The listing builds one solid part. Answer for the finished solid, in the listing's coordinates (mm). A direction names the side the tool comes from. Coordinates: 2 decimals unless noted, no trailing zeros. Order: outer loops, then holes, each group sorted by start corner. A loop starts at its lowest first (then second) coordinate and runs counter-clockwise, first axis right, second up. Notation, with made-up numbers: (41.25, 83) -> (82.25, 83) arc R9 ccw to (82.25, 92) -> close; hole circle Ø3 at (78.5, 25). An arc over 180 degrees is marked (long way). Write item = value, one per line. Start each with the question number.
Autodesk Inventor part; units mm, degrees
ref_plane "Work Plane1" through (0, 0, -10) normal (0, 0, 1) x (1, 0, 0)
ref_plane "Work Plane2" through (0, 0, 0) normal (0.7071, -0.7071, 0) x (0, 0, -1)
ref_plane "YZ Plane" through (0, 0, 0) normal (1, 0, 0) x (0, 1, 0)
sketch "Sketch1" plane through (0, 0, 0) normal (0, 0, 1) x (1, 0, 0)
  line L0 (0, 0) -> (27.5, 0)
  line L1 (27.5, 0) -> (27.5, 5.5)
  line L2 (27.5, 5.5) -> (23, 5.5)
  line L3 (0, 0) -> (0, 27.5)
  line L4 (0, 0) -> (27.5, 0) construction
  line L5 (0, 27.5) -> (5.5, 27.5)
  line L6 (5.5, 27.5) -> (5.5, 23)
  line L7 (5.5, 23) -> (23, 5.5)
  dimension "d0" = 27.5
  dimension "d1" = 5.5
  dimension "d2" = 4.5
  dimension "d3" = 27.5
  dimension "d4" = 90
  dimension "d5" = 5.5
  dimension "d6" = 4.5
sketch "Sketch2" plane through (0, 0, 0) normal (0, 0, 1) x (1, 0, 0)
  line L0 (0, 0) -> (3.5, 0)
  line L1 (3.5, 3.5) -> (3.5, 27.5)
  line L2 (3.5, 27.5) -> (0, 27.5)
  line L3 (0, 27.5) -> (0, 0)
  line L4 (0, 0) -> (27.5, 0)
  line L5 (27.5, 0) -> (27.5, 3.5)
  line L6 (27.5, 3.5) -> (3.5, 3.5)
  line L7 (0, 3.5) -> (0, 0)
  dimension "d7" = 3.5
  dimension "d8" = 27.5
  dimension "d9" = 27.5
  dimension "d10" = 3.5
extrude "Extrusion1" add sketch "Sketch2" against normal blind 20
extrude "Extrusion2" add sketch "Sketch1" against normal blind 3.5
ref_plane "Work Plane1" through (0, 0, -10) normal (0, 0, 1) x (1, 0, 0)
mirror "Mirror1" about plane through (0, 0, -10) normal (0, 0, 1) of "Extrusion2"
sketch "Sketch3" plane through (0, 0, 0) normal (-1, 0, 0) x (0, 0, 1)
  line L0 (0, 0) -> (-20, 0) construction
  line L1 (-10, 0) -> (-10, 15) construction
  line L2 (-10, 14.8275) -> (-6.75, 14.8275) construction
  line L3 (-6.75, 14.8275) -> (-6.75, 9.8275) construction
  line L4 (-10, 9.8275) -> (-10, 14.8275) construction
  line L5 (-13.25, 13.0775) -> (-13.25, 17.1562)
  line L6 (-10, 20.4062) -> (-10, 20.4062)
  line L7 (-6.75, 17.1562) -> (-6.75, 13.0775)
  arc A0 (-10, 20.4062) -> (-13.25, 17.1562) centre (-10, 17.1562) ccw
  arc A1 (-6.75, 17.1562) -> (-10, 20.4062) centre (-10, 17.1562) ccw
  arc A2 (-13.25, 13.0775) -> (-10, 9.8275) centre (-10, 13.0775) ccw
  line L8 (-10, 9.8275) -> (-10, 9.8275)
  arc A3 (-10, 9.8275) -> (-6.75, 13.0775) centre (-10, 13.0775) ccw
  point P0 (-13.25, 20.4062)
  point P1 (-6.75, 20.4062)
  dimension "d16" = 15
  dimension "d17" = 3.25
  dimension "d18" = 5
  dimension "d19" = 6.5
  dimension "d20" = 3.25
  dimension "d21" = 3.25
extrude "Extrusion3" cut sketch "Sketch3" against normal through all
ref_plane "Work Plane2" through (0, 0, 0) normal (0.7071, -0.7071, 0) x (0, 0, -1)
mirror "Mirror2" about plane through (0, 0, 0) normal (0.7071, -0.7071, 0) of "Extrusion3"
properties part number "bracket"
Item 1: Consider probe 1 along Z at (x, y) = (4.5, 15.25); probe 2 along X at (y, z) = (25.75, -8.5). Determine where each line is inside the solid, lowest interval first.
Item 2: Section C-C, the plane x = 8.5 is taken. Give the vertices of the cut face in (y, z), then the cut area to 4 significant figures.
Item 3: Section B-B, the plane y = 16 is taken. Give the vertices of the cut face in (x, z).
Item 4: Each of these flat-tipped pins is pushed along its axis until it touches: pin 1 (6 mm diameter, centred on y = 9, z = -11.5, fed in from +X); pin 2 (5 mm diameter, centred on x = 9, z = -8.5, fed in from +Y); pin 3 (1.8 mm diameter, centred on x = 26, z = -19, fed in from +Y). Where does it stop, or does it pass through?
Item 5: Which of the six approach directions +Z, -Z, +X, -X, +Y, -Y give full straight-line access (tool end or side, diameter ignored) to faces 1 (the flat face through (5.5, 25, -2)), 2 (the flat face through (11, 11, 0)), 3 (the flat face through (10, 10, -3.5)), 4 (the cylindrical face through (1.73, 9.83, -10.07)), 5 (the flat face through (15, 2, -6.75))?
Item 6: Section D-D, the plane y = 23.75 is taken. Give the vertices of the cut face in (x, z), then the cut area to 3 significant figures.
Item 7: For a pull along Y with two mould halves and no side action, classify faces 6 (the flat face through (16, 3.5, -6)), 7 (the flat face through (2, 15, -6.75)), 8 (the flat face through (11, 11, -20)) as pulls with the +Y half, pulls with the -Y half, needs draft (parallel to the pull), parting line crosses it, or undercut.
Item 8: Section A-A, the plane z = -10 is taken. Give the vertices of the cut face in (x, y).
A:
q1.probe_1 = -20 to -16.5, -3.5 to 0
q1.probe_2 = 0 to 3.5
q2.outline = (0, -20) -> (20, -20) -> (20, -16.5) -> (3.5, -16.5) -> (3.5, -3.5) -> (20, -3.5) -> (20, 0) -> (0, 0) -> close
q2.area = 185.5 mm^2
q3.outline = (0, -20) -> (12.5, -20) -> (12.5, -16.5) -> (3.5, -16.5) -> (3.5, -13.25) -> (0, -13.25) -> close; (0, -6.75) -> (3.5, -6.75) -> (3.5, -3.5) -> (12.5, -3.5) -> (12.5, 0) -> (0, 0) -> close
q4.pin_1 = 3.5
q4.pin_2 = 3.5
q4.pin_3 = 5.5
q5.face_1 = +Z, -Z, +X, +Y
q5.face_2 = +Z, +X, -X, +Y, -Y
q5.face_3 = +X, +Y
q5.face_4 = +X, -X
q5.face_5 = +Y, -Y
q6.outline = (0, -20) -> (5.5, -20) -> (5.5, -16.5) -> (3.5, -16.5) -> (3.5, -3.5) -> (5.5, -3.5) -> (5.5, 0) -> (0, 0) -> close
q6.area = 84.0 mm^2
q7.face_6 = pulls with the +Y half
q7.face_7 = undercut
q7.face_8 = needs draft
q8.outline = (0, 0) -> (9.83, 0) -> (9.83, 3.5) -> (3.5, 3.5) -> (3.5, 9.83) -> (0, 9.83) -> close; (0, 20.41) -> (3.5, 20.41) -> (3.5, 27.5) -> (0, 27.5) -> close; (20.41, 0) -> (27.5, 0) -> (27.5, 3.5) -> (20.41, 3.5) -> close
